Check sheet for the modelled part. Datum: model origin and axes. Units: mm. Face numbers are marked on the shaded views. Round coordinates to 2 decimals unless told otherwise and drop trailing zeros. Write each loop counter-clockwise with the first axis right and the second up, starting at its lowest first coordinate (ties: lowest second). Pieces come first, ordered by that corner, then holes.
Item 1: Cross-section at A-A on x = 0. Enter the section's corners in (y, z).
Item 2: Go/stop test with flat-tipped pins: pin 1 Ø8 at (x, y) = (120, -9.5) entering from -Z; pin 2 Ø1 at (x, z) = (44.5, 29.5) entering from -Y; pin 3 Ø2 at (x, z) = (149.5, 17.5) entering from +Y; pin 4 Ø8 at (x, y) = (155, -0.5) entering from -Z. Record where each tip stops, or that it passes through.
Item 3: Material ranges on line 1 (X direction, y = -2, z = 8.5); line 2 (X direction, y = -13, z = 0); line 3 (X direction, y = -1, z = 0), recorded low to high.
Item 4: Cross-section at D-D on x = 170. Enter the section's corners in (y, z).
Item 5: Release check for a two-part mould opening along Z. For the marked faces 1 and 2 record: +Z half, -Z half, draft (parallel to the pull), parting line (faces both ways), or undercut.
Item 6: Cross-section at C-C on y = -16.5. Enter the section's corners in (x, z).
Item 7: Cross-section at B-B on z = 34.5. Enter the section's corners in (x, y), plus the area to 3 significant figures.
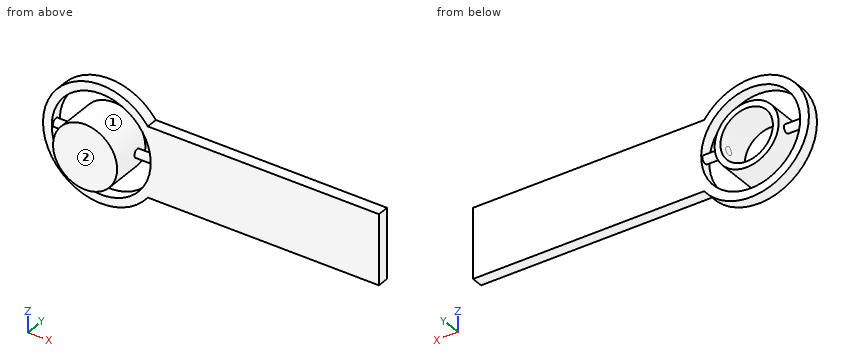
from build123d import *

# Parameters (mm, degrees)
EXTRUDE_THIN1_DEPTH      = 10
EXTRUDE_THIN1_DEPTH_BACK = 25
SKETCH1_R                = 27.5
SKETCH1_R_2              = 22.5
SKETCH3_R                = 22.5
BOSS_EXTRUDE1_DEPTH      = 5
BOSS_EXTRUDE2_DEPTH      = 5
BOSS_EXTRUDE2_DEPTH_BACK = 5
SKETCH1_4_R              = 50
SKETCH1_4_R_2            = 42.5
CUT_EXTRUDE1_REACH       = 220.167
CUT_EXTRUDE1_END_RADIUS  = 22.5
SKETCH5_R                = 3.5
BOSS_EXTRUDE3_REACH      = 205.704
BOSS_EXTRUDE3_END_RADIUS = 22.5
SKETCH6_R                = 3.5
SKETCH7_R                = 3.5
BOSS_EXTRUDE5_DEPTH      = 20


with BuildPart() as part:
    # Sketch1 → Extrude-Thin1 (new, two sides: drawn at the far end of the back side and taken through both)
    with BuildSketch(Plane(origin=(0, 0, 0), x_dir=(1, 0, 0), z_dir=(0, 1, 0)).offset(-EXTRUDE_THIN1_DEPTH_BACK)):
        Circle(SKETCH1_R)
        Circle(SKETCH1_R_2, mode=Mode.SUBTRACT)
    extrude(amount=EXTRUDE_THIN1_DEPTH + EXTRUDE_THIN1_DEPTH_BACK)

    # Sketch3 → Boss-Extrude1 (add)
    with BuildSketch(Plane.XZ.offset(25)):
        with Locations(Location((0, 0, 0), (0, 0, 90))):
            Circle(SKETCH3_R)
    extrude(amount=-BOSS_EXTRUDE1_DEPTH)

    # Cut-Extrude1: up to this cylinder (the profile starts outside it)
    cut_extrude1_end = Plane(origin=(0, 0, 0), z_dir=(0, 1, 0)) * Cylinder(CUT_EXTRUDE1_END_RADIUS, 486.334, mode=Mode.PRIVATE)
    # Sketch5 → Cut-Extrude1 (cut, up to the surface)
    with BuildSketch(Plane(origin=(27.5, 0, 0), x_dir=(0, 0, -1), z_dir=(1, 0, 0)), mode=Mode.PRIVATE) as cut_extrude1_sk1:
        Circle(SKETCH5_R)
    cut_extrude1_tool1 = extrude(cut_extrude1_sk1.sketch, amount=-CUT_EXTRUDE1_REACH, mode=Mode.PRIVATE) - cut_extrude1_end
    cut_extrude1 = cut_extrude1_tool1.solids().sort_by_distance((27.5, 0, 0))[0]
    add(cut_extrude1, mode=Mode.SUBTRACT)

    # Mirror1: Cut-Extrude1 across plane
    add(cut_extrude1.mirror(Plane(origin=(0, 0, 0), x_dir=(0, 0, 1), z_dir=(1, 0, 0))), mode=Mode.SUBTRACT)



with BuildPart() as body_2:
    # Sketch1<4> → Boss-Extrude2 (new, two sides: drawn at the far end of the back side and taken through both)
    # profile 1 of 2: a face of its own
    with BuildSketch(Plane(origin=(0, 0, 0), x_dir=(1, 0, 0), z_dir=(0, 1, 0)).offset(-BOSS_EXTRUDE2_DEPTH_BACK)):
        Circle(SKETCH1_4_R)
        with Locations(Location((0, 0, 0), (0, 0, 270))):
            Circle(SKETCH1_4_R_2, mode=Mode.SUBTRACT)
    # profile 2 of 2: a face of its own
    with BuildSketch(Plane(origin=(0, 0, 0), x_dir=(1, 0, 0), z_dir=(0, 1, 0)).offset(-BOSS_EXTRUDE2_DEPTH_BACK)):
        with BuildLine():
            ThreePointArc((50, 0), (47.434164903, -15.811388301), (40, -30))
            Line((40, -30), (238.383087675, -30))
            Line((238.383087675, -30), (238.383087675, 30))
            Line((238.383087675, 30), (40, 30))
            ThreePointArc((40, 30), (47.434164903, 15.811388301), (50, 0))
        make_face()
    extrude(amount=BOSS_EXTRUDE2_DEPTH + BOSS_EXTRUDE2_DEPTH_BACK)


with BuildPart() as part_1:
    add(part.part)

    add(body_2.part)  # Boss-Extrude3 merges body 2
    # Boss-Extrude3: up to this cylinder (the profile starts outside it)
    boss_extrude3_end = Plane(origin=(0, 0, 0), z_dir=(0, 1, 0)) * Cylinder(BOSS_EXTRUDE3_END_RADIUS, 457.408, mode=Mode.PRIVATE)
    # Sketch6 → Boss-Extrude3 (add, up to the surface)
    with BuildSketch(Plane.ZY.offset(-42.5), mode=Mode.PRIVATE) as boss_extrude3_sk1:
        with Locations(Location((0, 0, 0), (0, 0, 180))):
            Circle(SKETCH6_R)
    boss_extrude3_tool1 = extrude(boss_extrude3_sk1.sketch, amount=BOSS_EXTRUDE3_REACH, mode=Mode.PRIVATE) - boss_extrude3_end
    add(boss_extrude3_tool1.solids().sort_by_distance((42.5, 0, 0))[0])

    # Sketch7 → Boss-Extrude5 (add)
    with BuildSketch(Plane(origin=(-42.5, 0, 0), x_dir=(0, 0, -1), z_dir=(1, 0, 0))):
        Circle(SKETCH7_R)
    extrude(amount=BOSS_EXTRUDE5_DEPTH)


solid = part_1.part
Response values:
1. outline: (-25, -27.5) - (10, -27.5) - (10, -22.5) - (-20, -22.5) - (-20, 22.5) - (10, 22.5) - (10, 27.5) - (-25, 27.5) - close; (-5, -50) - (5, -50) - (5, -42.5) - (-5, -42.5) - close; (-5, 42.5) - (5, 42.5) - (5, 50) - (-5, 50) - close
2. pin 1: passes through
2. pin 2: stops at y = -5
2. pin 3: stops at y = 5
2. pin 4: stops at z = -30
3. line 1: x = -49.27 to -41.64, -26.15 to -20.83, 20.83 to 26.15, 41.64 to 238.38
3. line 2: x = -27.5 to -22.5, 22.5 to 27.5
3. line 3: x = -50 to -22.5, 22.5 to 238.38
4. outline: (-5, -30) - (5, -30) - (5, 30) - (-5, 30) - close
5. face 1: undercut
5. face 2: draft
6. outline: circle Ø55 at (0, 0); hole circle Ø45 at (0, 0)
7. outline: (-36.19, -5) - (-24.82, -5) - (-24.82, 5) - (-36.19, 5) - close; (24.82, -5) - (36.19, -5) - (36.19, 5) - (24.82, 5) - close
7. area: 227 mm2
